Check sheet for the drawn part. Datum: minimum x, y, z corner. Units: mm. A direction names the side the tool comes from. Coordinates: 2 decimals unless noted, no trailing zeros. Loops run counter-clockwise (first coordinate to the right, second up) from the corner with the lowest first, then second, coordinate; pieces in that order, holes last. Notation, with made-up numbers: (-7, -39) - (-1, -39) arc R6 cw to (-1, -32) - close; hole circle Ø5 at (3, 72). An arc over 180 degrees is marked (long way). Answer as CSV lines item,"result". Start each with the question number.
1. Set-up check for the marked faces 1 and 2: record each of +Z, -Z, +X, -X, +Y, -Y from which the full face is reachable in a straight line by a thin tool's end or side.
2. Cross-section at B-B (y = 5.5). Enter the section's corners in (x, z).
3. Cross-section at D-D (z = 7.5). Enter the section's corners in (x, y), plus the area to 3 significant figures.
4. Gauge pin test, flat ends, axial feed: P1, Ø4, axis at x = 22.5, y = 6, coming from the -Z side; P2, Ø10, axis at x = 28.5, z = 42.5, coming from the +Y side; P3, Ø1.1, axis at y = 0.5, z = 14, coming from the -X side; P4, Ø4, axis at x = 31.5, z = 53, coming from the -Y side. Record the tip position at first contact, or that the pin passes through.
5. Material ranges on line 1 (X direction, y = 1.25, z = 36.5); line 2 (X direction, y = 10.5, z = 57); line 3 (Z direction, x = 38, y = 14), recorded low to high. Write a range as [from, to].
6. Cross-section at A-A (z = 60). Enter the section's corners in (x, y), plus the area to 3 significant figures.
7. Cross-section at C-C (x = 42.5). Enter the section's corners in (y, z), plus the area to 3 significant figures.
8. Release check for a two-part mould opening along X. For the marked faces 3, 4, 5 and 6 record: pulls with the +X half, pulls with the -X half, needs draft (parallel to the pull), parting line crosses it, or undercut.
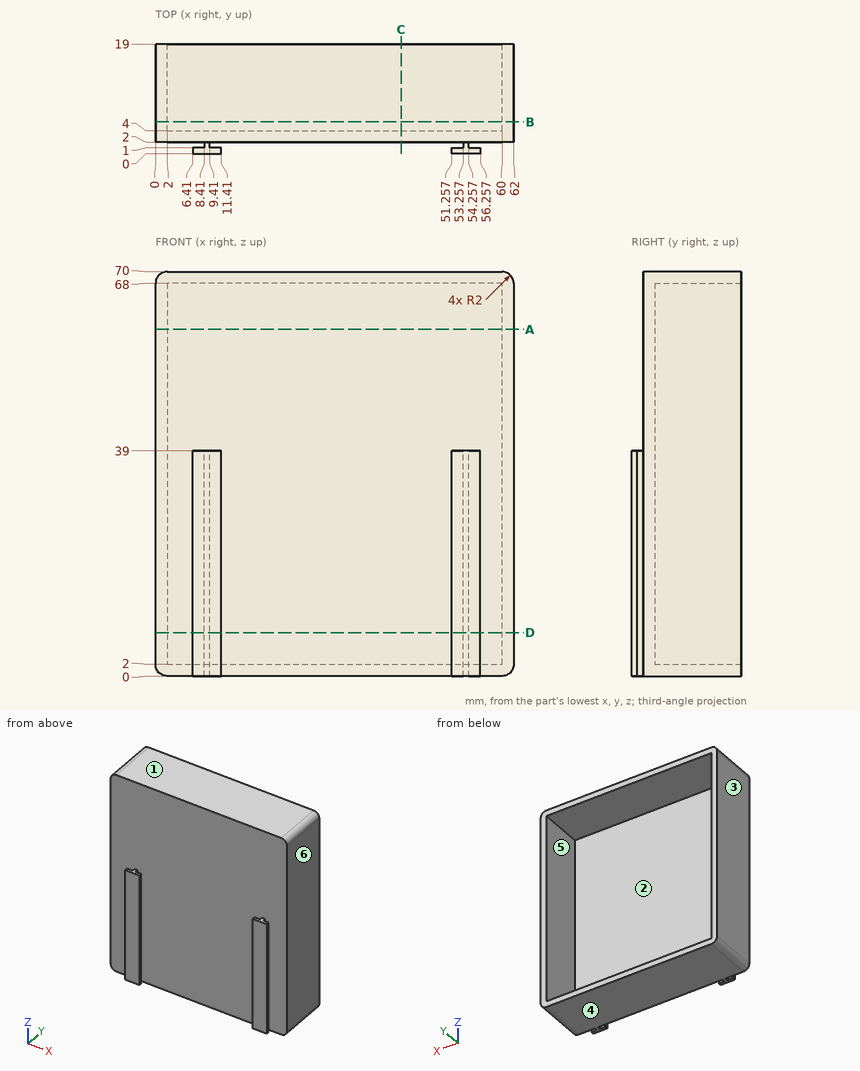
Values follow:
1,face 1,"+Z, +X, -X, +Y, -Y"
1,face 2,"+Y"
2,outline,"(0, 2) arc R2 ccw to (2, 0) - (60, 0) arc R2 ccw to (62, 2) - (62, 68) arc R2 ccw to (60, 70) - (2, 70) arc R2 ccw to (0, 68) - close; hole (2, 2) - (60, 2) - (60, 68) - (2, 68) - close"
3,outline,"(0, 2) - (8.41, 2) - (8.41, 1) - (6.41, 1) - (6.41, 0) - (11.41, 0) - (11.41, 1) - (9.41, 1) - (9.41, 2) - (53.26, 2) - (53.26, 1) - (51.26, 1) - (51.26, 0) - (56.26, 0) - (56.26, 1) - (54.26, 1) - (54.26, 2) - (62, 2) - (62, 19) - (60, 19) - (60, 4) - (2, 4) - (2, 19) - (0, 19) - close"
3,area,"196 mm²"
4,P1,"stops at z = 0"
4,P2,"stops at y = 4"
4,P3,"stops at x = 6.41"
4,P4,"stops at y = 2"
5,line 1,"x = [8.41, 9.41], [53.26, 54.26]"
5,line 2,"x = [0, 2], [60, 62]"
5,line 3,"z = [0, 2], [68, 70]"
6,outline,"(0, 2) - (62, 2) - (62, 19) - (60, 19) - (60, 4) - (2, 4) - (2, 19) - (0, 19) - close"
6,area,"184 mm²"
7,outline,"(2, 0) - (19, 0) - (19, 2) - (4, 2) - (4, 68) - (19, 68) - (19, 70) - (2, 70) - close"
7,area,"200 mm²"
8,face 3,"pulls with the -X half"
8,face 4,"needs draft"
8,face 5,"undercut"
8,face 6,"pulls with the +X half"
